Part print with two shaded views. Sizes in mm from the minimum x, y, z corner. A direction names the side the tool comes from. Coordinates: 2 decimals unless noted, no trailing zeros. Write each loop counter-clockwise with the first axis right and the second up, starting at its lowest first coordinate (ties: lowest second). Pieces come first, ordered by that corner, then holes. Notation, with made-up numbers: M 64,18.25 L 70,18.25 A12 ccw 70,25.25 Z; hole C -19,-17.75 d6. An arc over 180 degrees is marked long. Answer in a Markdown table with one row per item. Add a question column.
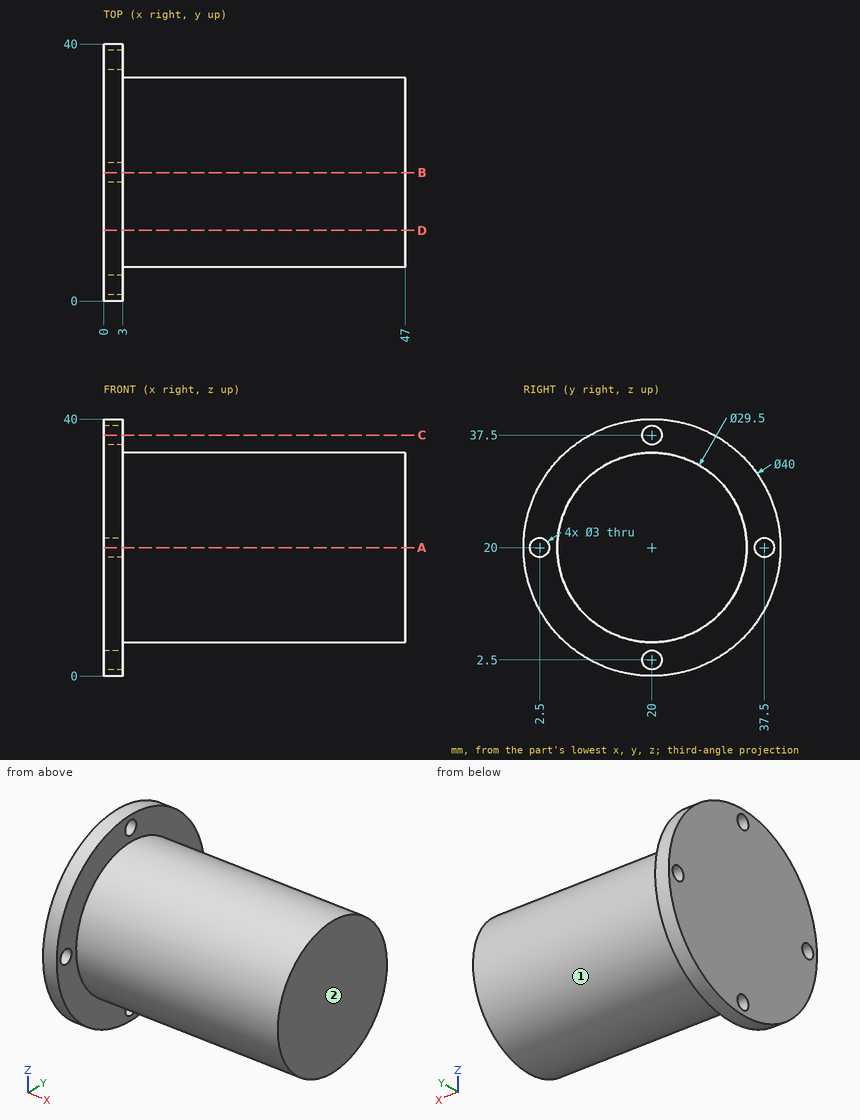
1) Slice it at A-A (z = 20). Give the cut face in (x, y), then the cut area to 3 significant figures.
2) Slice it at C-C (z = 37.5). Give the cut face in (x, y).
3) Slice it at D-D (y = 11). Give the cut face in (x, z), then the cut area to 3 significant figures.
4) Drill centre lines: probe 1 along Y at (x, z) = (2.1, 20); probe 2 along Z at (x, y) = (2.5, 32); probe 3 along X at (y, z) = (27, 37.5). Where is each one in solid material? Low to high.
5) Which spindle directions (+Z, -Z, +X, -X, +Y, -Y) get a long thin tool onto all of the face, cutting with end or side? Do the marked faces 1 and 2. Say none if no direction does.
6) Flat gauge pins, fed straight in: pin 1 Ø10 at (x, z) = (24.5, 16) entering from +Y; pin 2 Ø5 at (x, y) = (28.5, 26.5) entering from +Z; pin 3 Ø8 at (x, z) = (17.5, 21.5) entering from -Y; pin 4 Ø2.5 at (y, z) = (20, 37.5) entering from -X. Where does each tip first touch, or does it go through?
Ans:
| question | item | result |
|---|---|---|
| 1 | outline | M 0,0 L 3,0 L 3,1 L 0,1 Z; M 0,4 L 3,4 L 3,5.25 L 47,5.25 L 47,34.75 L 3,34.75 L 3,36 L 0,36 Z; M 0,39 L 3,39 L 3,40 L 0,40 Z |
| 1 | area | 1,400 mm2 |
| 2 | outline | M 0,10.32 L 3,10.32 L 3,18.5 L 0,18.5 Z; M 0,21.5 L 3,21.5 L 3,29.68 L 0,29.68 Z |
| 3 | outline | M 0,2.14 L 3,2.14 L 3,8.31 L 47,8.31 L 47,31.69 L 3,31.69 L 3,37.86 L 0,37.86 Z |
| 3 | area | 1,140 mm2 |
| 4 | probe 1 | y = 0 to 1, 4 to 36, 39 to 40 |
| 4 | probe 2 | z = 4 to 36 |
| 4 | probe 3 | x = 0 to 3 |
| 5 | face 1 | +X |
| 5 | face 2 | +Z, -Z, +X, +Y, -Y |
| 6 | pin 1 | stops at y = 34.75 |
| 6 | pin 2 | stops at z = 34.2 |
| 6 | pin 3 | stops at y = 5.25 |
| 6 | pin 4 | passes through |
